For this review, take the finished solid that the model builds, in its own axes (mm). A direction names the side the tool comes from. Round coordinates to 2 decimals unless told otherwise and drop trailing zeros. Loops run counter-clockwise (first coordinate to the right, second up) from the corner with the lowest first, then second, coordinate; pieces in that order, holes last. Notation, with made-up numbers: (70.5, 4.5) -> (107.5, 4.5) arc R18 cw to (107.5, 11.5) -> close; hole circle Ø11 at (4, 69.25). An arc over 180 degrees is marked (long way). Write each question's results on one line, items separated by ' | '.
```python
from build123d import *

# Parameters (mm, degrees)
RESSALTO_EXTRUS_O1_DEPTH   = 7.5
ESBO_O2_R                  = 11
RESSALTO_EXTRUS_O2_DEPTH   = 11
RESSALTO_EXTRUS_O4_DEPTH   = 2.5
RESSALTO_EXTRUS_O5_DEPTH   = 7.5
ESBO_O5_R                  = 7.5
RESSALTO_EXTRUS_O6_DEPTH   = 6
ESBO_O6_W                  = 21
ESBO_O6_H                  = 7
CORTE_EXTRUS_O1_DEPTH      = 88.647057938
CORTE_EXTRUS_O3_DEPTH      = 92.969424267
CORTE_EXTRUS_O3_DEPTH_BACK = 92.969424267
ESBO_O7_R                  = 3.5
CORTE_EXTRUS_O5_DEPTH      = 92.969424267
CORTE_EXTRUS_O5_DEPTH_BACK = 92.969424267
ESBO_O8_R                  = 7.5
CORTE_EXTRUS_O6_DEPTH      = 87.070855116
CORTE_EXTRUS_O6_DEPTH_BACK = 87.070855116
ESBO_O9_R                  = 3.5


with BuildPart() as part:
    # Esbo_o1 → Ressalto-extrus_o1 (new, symmetric)
    with BuildSketch(Plane.XY):
        with BuildLine():
            Line((-65, 7.5), (-50, 7.5))
            Line((-50, 7.5), (-50, -7.5))
            Line((-50, -7.5), (-65, -7.5))
            ThreePointArc((-65, -7.5), (-72.5, 0), (-65, 7.5))
        make_face()
    extrude(amount=RESSALTO_EXTRUS_O1_DEPTH, both=True)



with BuildPart() as body_2:
    # Esbo_o2 → Ressalto-extrus_o2 (new, symmetric)
    with BuildSketch(Plane.XY):
        Circle(ESBO_O2_R)
    extrude(amount=RESSALTO_EXTRUS_O2_DEPTH, both=True)


with BuildPart() as part_1:
    add(part.part)

    add(body_2.part)  # Ressalto-extrus_o4 merges body 2
    # Esbo_o3 → Ressalto-extrus_o4 (add, symmetric)
    with BuildSketch(Plane.XY):
        Polygon((-50, 7.5), (0, 11), (0, -11), (-50, -7.5), align=None)
    extrude(amount=RESSALTO_EXTRUS_O4_DEPTH, both=True)

    # Esbo_o4 → Ressalto-extrus_o5 (add, symmetric)
    with BuildSketch(Plane.XY):
        Polygon((2.121320344, -2.121320344), (48.083261121, 43.840620434), (43.840620434, 48.083261121), (-2.121320344, 2.121320344), align=None)
    extrude(amount=RESSALTO_EXTRUS_O5_DEPTH, both=True)

    # Esbo_o5 → Ressalto-extrus_o6 (add, symmetric)
    with BuildSketch(Plane(origin=(0, 0, 0), x_dir=(0, 0, 1), z_dir=(-0.7071067811865488, 0.7071067811865464, 0))):
        with Locations(Location((0, 65, 0), (0, 0, 270))):
            Circle(ESBO_O5_R)
    extrude(amount=RESSALTO_EXTRUS_O6_DEPTH, both=True)

    # Esbo_o6 → Corte-extrus_o1 (cut, through all)
    with BuildSketch(Plane(origin=(0, 7.5, 0), x_dir=(1, 0, 0), z_dir=(0, 1, 0))):
        with Locations((-65, 0)):
            Rectangle(ESBO_O6_W, ESBO_O6_H)
    extrude(amount=-CORTE_EXTRUS_O1_DEPTH, mode=Mode.SUBTRACT)

    # Esbo_o7 → Corte-extrus_o3 (cut, two sides: drawn at the far end of the back side and taken through both)
    with BuildSketch(Plane.XY.offset(-CORTE_EXTRUS_O3_DEPTH_BACK)):
        with Locations((-65, 0)):
            Circle(ESBO_O7_R)
    extrude(amount=CORTE_EXTRUS_O3_DEPTH + CORTE_EXTRUS_O3_DEPTH_BACK, mode=Mode.SUBTRACT)

    # Esbo_o8 → Corte-extrus_o5 (cut, two sides: drawn at the far end of the back side and taken through both)
    with BuildSketch(Plane.XY.offset(-CORTE_EXTRUS_O5_DEPTH_BACK)):
        Circle(ESBO_O8_R)
    extrude(amount=CORTE_EXTRUS_O5_DEPTH + CORTE_EXTRUS_O5_DEPTH_BACK, mode=Mode.SUBTRACT)

    # Esbo_o9 → Corte-extrus_o6 (cut, two sides: drawn at the far end of the back side and taken through both)
    with BuildSketch(Plane(origin=(-4.242640687, 4.242640687, 0), x_dir=(0, 0, 1), z_dir=(-0.7071067811865487, 0.7071067811865465, 0)).offset(-CORTE_EXTRUS_O6_DEPTH_BACK)):
        with Locations(Location((0, 65, 0), (0, 0, 270))):
            Circle(ESBO_O9_R)
    extrude(amount=CORTE_EXTRUS_O6_DEPTH + CORTE_EXTRUS_O6_DEPTH_BACK, mode=Mode.SUBTRACT)


solid = part_1.part
```
1. Draft analysis for pull direction X (two halves, no side actions). For faces 5 (the face through (-61, 0, 7.5)), 6 (the face through (-72.5, -0.16, -5.47)), 7 (the face through (-68.497, 0.154, -5.528)), state which applies: released by +X, released by -X, zero draft, split by the parting line, or undercut.
Values found:
face 5: zero draft | face 6: released by -X | face 7: undercut
2. Consider section A-A (z = -5). State the section outline as (x, y) points, plus the area to 3 significant figures.
Values found:
outline: (-65, -7.5) -> (-50, -7.5) -> (-50, 7.5) -> (-65, 7.5) arc R7.5 ccw to start; (5.36, 9.6) arc R11 ccw (long way) to (9.6, 5.36) -> (44.13, 39.89) -> (46.25, 37.77) -> (54.16, 45.67) -> (45.67, 54.16) -> (37.77, 46.25) -> (39.89, 44.13) -> close; hole circle Ø7 at (-65, 0); hole circle Ø15 at (0, 0) | area: 904 mm2
3. Consider section B-B (x = -56.5). State the section outline as (y, z) points.
Values found:
outline: (-7.5, -7.5) -> (7.5, -7.5) -> (7.5, -3.5) -> (-7.5, -3.5) -> close; (-7.5, 3.5) -> (7.5, 3.5) -> (7.5, 7.5) -> (-7.5, 7.5) -> close
4. To check wall thickness, follow probe 1 along X at (y, z) = (0, 1.25); probe 2 along Z at (x, y) = (-56.5, 1.5); probe 3 along Y at (x, z) = (0, 5.5). State the ranges of each line that lie inside material, in increasing order.
Values found:
probe 1: x = -54.5 to -7.5, 7.5 to 11 | probe 2: z = -7.5 to -3.5, 3.5 to 7.5 | probe 3: y = -11 to -7.5, 7.5 to 11
5. For pin 1 (21.5 mm diameter, centred on x = 32.5, y = 28.5, fed in from +Z); pin 2 (1 mm diameter, centred on y = -0.5, z = -1.5, fed in from -X); pin 3 (1.5 mm diameter, centred on x = 31, z = -3, fed in from +Y); pin 4 (19.5 mm diameter, centred on x = 0, y = 0, fed in from -Z), all flat-tipped, find the tip position at first contact; note any pin that passes through.
Values found:
pin 1: stops at z = 7.5 | pin 2: stops at x = -54.5 | pin 3: stops at y = 35.99 | pin 4: stops at z = -11
6. Consider section C-C (y = 0). State the section outline as (x, z) points.
Values found:
outline: (-72.5, -7.5) -> (-68.5, -7.5) -> (-68.5, -3.5) -> (-72.5, -3.5) -> close; (-72.5, 3.5) -> (-68.5, 3.5) -> (-68.5, 7.5) -> (-72.5, 7.5) -> close; (-61.5, -7.5) -> (-50, -7.5) -> (-50, -2.5) -> (-11, -2.5) -> (-11, -11) -> (-7.5, -11) -> (-7.5, 11) -> (-11, 11) -> (-11, 2.5) -> (-50, 2.5) -> (-50, 7.5) -> (-61.5, 7.5) -> (-61.5, 3.5) -> (-54.5, 3.5) -> (-54.5, -3.5) -> (-61.5, -3.5) -> close; (7.5, -11) -> (11, -11) -> (11, 11) -> (7.5, 11) -> close
7. Consider section D-D (z = 5.75). State the section outline as (x, y) points.
Values found:
outline: (-65, -7.5) -> (-50, -7.5) -> (-50, 7.5) -> (-65, 7.5) arc R7.5 ccw to start; (5.36, 9.6) arc R11 ccw (long way) to (9.6, 5.36) -> (44.68, 40.44) -> (46.8, 38.31) -> (53.61, 45.12) -> (45.12, 53.61) -> (38.31, 46.8) -> (40.44, 44.68) -> close; hole circle Ø7 at (-65, 0); hole circle Ø15 at (0, 0)
8. Tool access review of faces 1 (the face through (-61.6, 1.8, -3.5)), 2 (the face through (-61, 0, -7.5)), 3 (the face through (-54, 7.5, 0)), 4 (the face through (5.076, -9.759, 0.154)): name each direction out of +Z, -Z, +X, -X, +Y, -Y from which nothing blocks a thin tool from reaching the whole face with its end or side.
Values found:
face 1: -X, +Y, -Y | face 2: -Z, -X, +Y, -Y | face 3: +Z, -Z, -X, +Y | face 4: none
